Here's how the part is built. I have some questions about the finished solid (model axes, mm). A direction names the side the tool comes from. Give positions to 0.01 mm unless a question says otherwise; leave off trailing zeros. Write each loop counter-clockwise with the first axis right and the second up, starting at its lowest first coordinate (ties: lowest second). Pieces come first, ordered by that corner, then holes. Notation, with made-up numbers: (80.25, -1) -> (117.25, -1) arc R25 ccw to (117.25, 13) -> close; hole circle Ø4 at (45.5, 59.25). An arc over 180 degrees is marked (long way). Use one line per item in the form item = value.
```python
from build123d import *

# Parameters (mm, degrees)
ESBO_O1_R                = 2
ESBO_O1_R_2              = 1.5
RESSALTO_EXTRUS_O1_DEPTH = 6
RESSALTO_EXTRUS_O2_START = -6
ESBO_O2_R                = 2
RESSALTO_EXTRUS_O2_DEPTH = 6
RESSALTO_EXTRUS_O4_DEPTH = 6


with BuildPart() as part:
    # Esboço1 → Ressalto-extrusão1 (new body)
    with BuildSketch(Plane(origin=(0, 0, 0), x_dir=(1, 0, 0), z_dir=(0, 1, 0))):
        with BuildLine():
            Line((99.9745166, -4.5254834), (71.398066402, 24.050966799))
            Line((71.398066402, 24.050966799), (-71.398066402, 24.050966799))
            Line((-71.398066402, 24.050966799), (-99.9745166, -4.5254834))
            ThreePointArc((-99.9745166, -4.5254834), (-109.0254834, -4.5254834), (-109.0254834, 4.5254834))
            Line((-109.0254834, 4.5254834), (-89.5, 24.050966799))
            Line((-89.5, 24.050966799), (-89.5, 39.050966799))
            Line((-89.5, 39.050966799), (-102.5, 52.050966799))
            Line((-102.5, 52.050966799), (-102.5, 86.949033201))
            Line((-102.5, 86.949033201), (-89.5, 99.949033201))
            Line((-89.5, 99.949033201), (-89.5, 109.050966799))
            Line((-89.5, 109.050966799), (-102.5, 122.050966799))
            Line((-102.5, 122.050966799), (-102.5, 156.949033201))
            Line((-102.5, 156.949033201), (-89.5, 169.949033201))
            Line((-89.5, 169.949033201), (-89.5, 184.949033201))
            Line((-89.5, 184.949033201), (-109.0254834, 204.4745166))
            ThreePointArc((-109.0254834, 204.4745166), (-109.0254834, 213.5254834), (-99.9745166, 213.5254834))
            Line((-99.9745166, 213.5254834), (-71.398066402, 184.949033201))
            Line((-71.398066402, 184.949033201), (71.398066402, 184.949033201))
            Line((71.398066402, 184.949033201), (99.9745166, 213.5254834))
            ThreePointArc((99.9745166, 213.5254834), (109.0254834, 213.5254834), (109.0254834, 204.4745166))
            Line((109.0254834, 204.4745166), (89.5, 184.949033201))
            Line((89.5, 184.949033201), (89.5, 169.949033201))
            Line((89.5, 169.949033201), (102.5, 156.949033201))
            Line((102.5, 156.949033201), (102.5, 122.050966799))
            Line((102.5, 122.050966799), (89.5, 109.050966799))
            Line((89.5, 109.050966799), (89.5, 99.949033201))
            Line((89.5, 99.949033201), (102.5, 86.949033201))
            Line((102.5, 86.949033201), (102.5, 52.050966799))
            Line((102.5, 52.050966799), (89.5, 39.050966799))
            Line((89.5, 39.050966799), (89.5, 24.050966799))
            Line((89.5, 24.050966799), (109.0254834, 4.5254834))
            ThreePointArc((109.0254834, 4.5254834), (109.0254834, -4.5254834), (99.9745166, -4.5254834))
        make_face()
        with Locations(Location((104.5, 209, 0), (0, 0, 270))):
            Circle(ESBO_O1_R, mode=Mode.SUBTRACT)
        with Locations(Location((104.5, 0, 0), (0, 0, 270))):
            Circle(ESBO_O1_R, mode=Mode.SUBTRACT)
        with Locations(Location((0, 125, 0), (0, 0, 270))):
            Circle(ESBO_O1_R_2, mode=Mode.SUBTRACT)
        with Locations(Location((0, 84, 0), (0, 0, 270))):
            Circle(ESBO_O1_R_2, mode=Mode.SUBTRACT)
        with Locations(Location((72.9, 139.5, 0), (0, 0, 270))):
            Circle(ESBO_O1_R_2, mode=Mode.SUBTRACT)
        with Locations(Location((92.9, 139.5, 0), (0, 0, 270))):
            Circle(ESBO_O1_R_2, mode=Mode.SUBTRACT)
        with Locations(Location((72.9, 69.5, 0), (0, 0, 270))):
            Circle(ESBO_O1_R_2, mode=Mode.SUBTRACT)
        with Locations(Location((92.9, 69.5, 0), (0, 0, 270))):
            Circle(ESBO_O1_R_2, mode=Mode.SUBTRACT)
        with Locations(Location((-92.9, 69.5, 0), (0, 0, 270))):
            Circle(ESBO_O1_R_2, mode=Mode.SUBTRACT)
        with Locations(Location((-72.9, 69.5, 0), (0, 0, 270))):
            Circle(ESBO_O1_R_2, mode=Mode.SUBTRACT)
        with Locations(Location((-92.9, 139.5, 0), (0, 0, 270))):
            Circle(ESBO_O1_R_2, mode=Mode.SUBTRACT)
        with Locations(Location((-72.9, 139.5, 0), (0, 0, 270))):
            Circle(ESBO_O1_R_2, mode=Mode.SUBTRACT)
        with Locations(Location((-104.5, 0, 0), (0, 0, 270))):
            Circle(ESBO_O1_R, mode=Mode.SUBTRACT)
        with Locations(Location((-104.5, 209, 0), (0, 0, 270))):
            Circle(ESBO_O1_R, mode=Mode.SUBTRACT)
        Polygon((-58.598066402, 172.149033201), (58.598066402, 172.149033201), (24.249033201, 137.8), (-24.249033201, 137.8), align=None, mode=Mode.SUBTRACT)
        Polygon((40.600966799, 136.05), (13.601933598, 109.050966799), (13.601933598, 99.949033201), (40.600966799, 72.95), (49.700966799, 72.95), (76.7, 99.949033201), (76.7, 109.050966799), (49.700966799, 136.05), align=None, mode=Mode.SUBTRACT)
        Polygon((-58.598066402, 36.850966799), (58.598066402, 36.850966799), (24.249033201, 71.2), (-24.249033201, 71.2), align=None, mode=Mode.SUBTRACT)
        Polygon((-40.600966799, 72.95), (-13.601933598, 99.949033201), (-13.601933598, 109.050966799), (-40.600966799, 136.05), (-49.700966799, 136.05), (-76.7, 109.050966799), (-76.7, 99.949033201), (-49.700966799, 72.95), align=None, mode=Mode.SUBTRACT)
    extrude(amount=RESSALTO_EXTRUS_O1_DEPTH)

    # Esboço2 → Ressalto-extrusão2 (add)
    with BuildSketch(Plane(origin=(0, 6, 0), x_dir=(1, 0, 0), z_dir=(0, 1, 0)).offset(RESSALTO_EXTRUS_O2_START)):
        with BuildLine():
            Line((-133.940126995, 228.040650721), (-9.918773353, 104.5))
            Line((-9.918773353, 104.5), (-133.940126995, -19.040650721))
            ThreePointArc((-133.940126995, -19.040650721), (-133.959349279, -28.940126995), (-124.059873005, -28.959349279))
            Line((-124.059873005, -28.959349279), (0, 94.619671505))
            Line((0, 94.619671505), (124.059873005, -28.959349279))
            ThreePointArc((124.059873005, -28.959349279), (133.959349279, -28.940126995), (133.940126995, -19.040650721))
            Line((133.940126995, -19.040650721), (9.918773353, 104.5))
            Line((9.918773353, 104.5), (133.940126995, 228.040650721))
            ThreePointArc((133.940126995, 228.040650721), (133.959349279, 237.940126995), (124.059873005, 237.959349279))
            Line((124.059873005, 237.959349279), (0, 114.380328495))
            Line((0, 114.380328495), (-124.059873005, 237.959349279))
            ThreePointArc((-124.059873005, 237.959349279), (-133.959349279, 237.940126995), (-133.940126995, 228.040650721))
        make_face()
        with Locations(Location((-129, 233, 0), (0, 0, 270))):
            Circle(ESBO_O2_R, mode=Mode.SUBTRACT)
        with Locations(Location((129, 233, 0), (0, 0, 270))):
            Circle(ESBO_O2_R, mode=Mode.SUBTRACT)
        with Locations(Location((129, -24, 0), (0, 0, 270))):
            Circle(ESBO_O2_R, mode=Mode.SUBTRACT)
        with Locations(Location((-129, -24, 0), (0, 0, 270))):
            Circle(ESBO_O2_R, mode=Mode.SUBTRACT)
        with Locations(Location((104.5, 0, 0), (0, 0, 270))):
            Circle(ESBO_O2_R, mode=Mode.SUBTRACT)
        with Locations(Location((-104.5, 0, 0), (0, 0, 270))):
            Circle(ESBO_O2_R, mode=Mode.SUBTRACT)
        with Locations(Location((104.5, 209, 0), (0, 0, 270))):
            Circle(ESBO_O2_R, mode=Mode.SUBTRACT)
        with Locations(Location((-104.5, 209, 0), (0, 0, 270))):
            Circle(ESBO_O2_R, mode=Mode.SUBTRACT)
    extrude(amount=RESSALTO_EXTRUS_O2_DEPTH)

    # Esboço4 → Ressalto-extrusão4 (add)
    with BuildSketch(Plane(origin=(0, 6, 0), x_dir=(1, 0, 0), z_dir=(0, 1, 0))):
        Polygon((102.5, 86.949033201), (110.840276613, 78.608756588), (110.840276613, 130.391243412), (102.5, 122.050966799), (102.5, 156.949033201), (110.840276613, 148.608756588), (110.840276613, 205.030334643), (122.88696922, 217.030334643), (122.88696922, -8.030334643), (110.840276613, 3.969665357), (110.840276613, 60.391243412), (102.5, 52.050966799), align=None)
        Polygon((-113.00671523, 226.949033201), (113.00671523, 226.949033201), (100.960022623, 214.949033201), (-100.960022623, 214.949033201), align=None)
        Polygon((-110.840276613, 130.391243412), (-110.840276613, 78.608756588), (-102.5, 86.949033201), (-102.5, 52.050966799), (-110.840276613, 60.391243412), (-110.840276613, 3.969665357), (-122.88696922, -8.030334643), (-122.88696922, 217.030334643), (-110.840276613, 205.030334643), (-110.840276613, 148.608756588), (-102.5, 156.949033201), (-102.5, 122.050966799), align=None)
        Polygon((-100.960022623, -5.949033201), (100.960022623, -5.949033201), (113.00671523, -17.949033201), (-113.00671523, -17.949033201), align=None)
    extrude(amount=-RESSALTO_EXTRUS_O4_DEPTH)


solid = part.part
```
Q1. I want a section at A-A, the plane z = -114. Write out the boundary of the cut face in (x, y), and give its area (3 significant figures).
Result set:
outline = (-122.89, 0) -> (-110.84, 0) -> (-110.84, 6) -> (-122.89, 6) -> close; (-94.45, 0) -> (-71.75, 0) -> (-71.75, 6) -> (-94.45, 6) -> close; (-19.46, 0) -> (19.46, 0) -> (19.46, 6) -> (-19.46, 6) -> close; (71.75, 0) -> (94.45, 0) -> (94.45, 6) -> (71.75, 6) -> close; (110.84, 0) -> (122.89, 0) -> (122.89, 6) -> (110.84, 6) -> close
area = 650 mm2
Q2. If I drill on line 1 along X through (y, z) = (4.95, -180); line 2 along X through (y, z) = (2.35, -122); line 3 along Z through (x, y) = (129, 2.8), over which ranges is the centre line in solid material (lowest first)? Write a range as from..to.
Result set:
line_1 = -122.89..-110.84, -89.5..89.5, 110.84..122.89
line_2 = -122.89..-110.84, -102.45..-63.75, -27.49..27.49, 63.75..102.45, 110.84..122.89
line_3 = -240..-235, -231..-223.12, 14.12..22, 26..31
Q3. I want a section at C-C, the plane y = 5.05. Count the separate pieces of the cut face and the enclosed holes in it, and give its area (3 significant figures).
Result set:
separate_pieces = 1
enclosed_holes = 30
area = 35,900 mm2
Q4. Which directions (+Z, -Z, +X, -X, +Y, -Y) give clear straight access to the entire face, cutting with the end or side of a thin tool? Please do faces 3 (the face through (128.49, 2.96, 13.61)), 4 (the face through (-128.34, 2.96, 13.46)), 5 (the face through (110.84, 3, -104)).
Result set:
face_3 = +X, +Y, -Y
face_4 = -X, +Y, -Y
face_5 = +Y, -Y
Q5. If we mould it in two halves opening along Z, with no side actions, what happens to faces 1 (the face through (-2, 3, -226.949)), 2 (the face through (46, 3, -136.05))? For each: +Z half, -Z half, draft (parallel to the pull), parting line (faces both ways), or undercut.
Result set:
face_1 = -Z half
face_2 = undercut
Q6. Will these pins go through, and if not, where does the flat tip stop? pin 1 Ø3 at (y, z) = (2, -32) entering from +X; pin 2 Ø1.8 at (y, z) = (4, -101.5) entering from -X.
Result set:
pin_1 = 122.89
pin_2 = -122.89
Q7. I want a section at B-B, the plane x = 67. Write out the boundary of the cut face in (y, z), and give its area (3 significant figures).
Result set:
outline = (0, -226.95) -> (6, -226.95) -> (6, -214.95) -> (0, -214.95) -> close; (0, -184.95) -> (6, -184.95) -> (6, -118.75) -> (0, -118.75) -> close; (0, -90.25) -> (6, -90.25) -> (6, -24.05) -> (0, -24.05) -> close; (0, 5.95) -> (6, 5.95) -> (6, 17.95) -> (0, 17.95) -> close
area = 938 mm2
Q8. I want a section at D-D, the plane x = -19. Write out the boundary of the cut face in (y, z).
Result set:
outline = (0, -226.95) -> (6, -226.95) -> (6, -214.95) -> (0, -214.95) -> close; (0, -184.95) -> (6, -184.95) -> (6, -172.15) -> (0, -172.15) -> close; (0, -137.8) -> (6, -137.8) -> (6, -113.55) -> (0, -113.55) -> close; (0, -95.45) -> (6, -95.45) -> (6, -71.2) -> (0, -71.2) -> close; (0, -36.85) -> (6, -36.85) -> (6, -24.05) -> (0, -24.05) -> close; (0, 5.95) -> (6, 5.95) -> (6, 17.95) -> (0, 17.95) -> close
